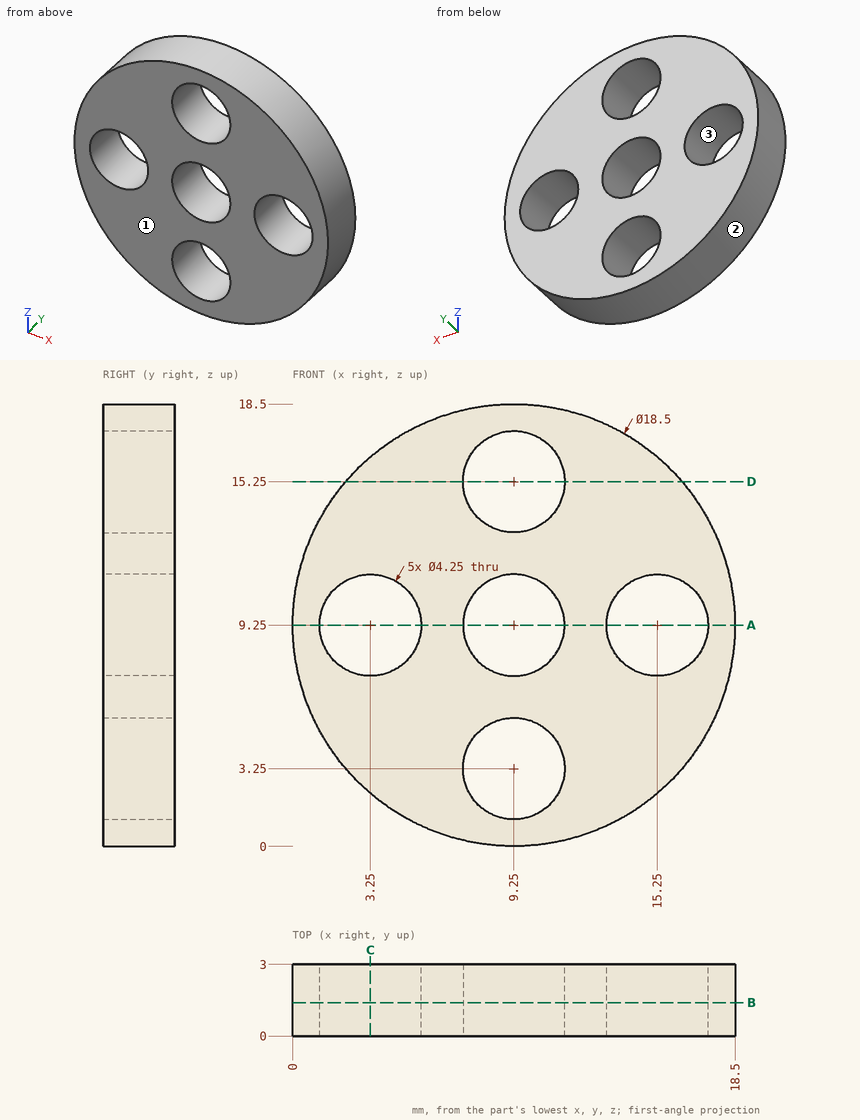
Can you work these out from the drawing? Everything is in mm from the part's minimum corner. Give positions to 0.01 mm unless a question says otherwise; leave off trailing zeros. Loops run counter-clockwise (first coordinate to the right, second up) from the corner with the lowest first, then second, coordinate; pieces in that order, holes last. Notation, with made-up numbers: (78, -15) -> (136, -15) arc R20 ccw to (136, 1) -> close; hole circle Ø5 at (61.25, 13). An arc over 180 degrees is marked (long way). Return JSON: item names as keys, results as strings.
Q1. I want a section at A-A, the plane z = 9.25. List the corners of the cut face in (x, y) for me (3 decimals), then the cut area to 4 significant figures.
Checks:
{"outline": "(0, 0) -> (1.125, 0) -> (1.125, 3) -> (0, 3) -> close; (5.375, 0) -> (7.125, 0) -> (7.125, 3) -> (5.375, 3) -> close; (11.375, 0) -> (13.125, 0) -> (13.125, 3) -> (11.375, 3) -> close; (17.375, 0) -> (18.5, 0) -> (18.5, 3) -> (17.375, 3) -> close", "area": "17.25 mm2"}
Q2. I want a section at C-C, the plane x = 3.25. List the corners of the cut face in (y, z) for me (3 decimals), then the cut area to 3 significant figures.
Checks:
{"outline": "(0, 2.21) -> (3, 2.21) -> (3, 7.125) -> (0, 7.125) -> close; (0, 11.375) -> (3, 11.375) -> (3, 16.29) -> (0, 16.29) -> close", "area": "29.5 mm2"}
Q3. I want a section at D-D, the plane z = 15.25. List the corners of the cut face in (x, y) for me (3 decimals), then the cut area to 3 significant figures.
Checks:
{"outline": "(2.21, 0) -> (7.125, 0) -> (7.125, 3) -> (2.21, 3) -> close; (11.375, 0) -> (16.29, 0) -> (16.29, 3) -> (11.375, 3) -> close", "area": "29.5 mm2"}
Q4. I want a section at B-B, the plane y = 1.4. List the corners of the cut face in (x, z) for me (3 decimals), then the cut area to 3 significant figures.
Checks:
{"outline": "circle Ø18.5 at (9.25, 9.25); hole circle Ø4.25 at (3.25, 9.25); hole circle Ø4.25 at (9.25, 3.25); hole circle Ø4.25 at (9.25, 9.25); hole circle Ø4.25 at (9.25, 15.25); hole circle Ø4.25 at (15.25, 9.25)", "area": "198 mm2"}
Q5. For pin 1 Ø5.5 at (x, z) = (3.25, 9.25) entering from +Y; pin 2 Ø2.5 at (x, z) = (9.25, 3.25) entering from -Y; pin 3 Ø1 at (y, z) = (2, 3.5) entering from +X, each with a flat end and sliding along its axis, tell me the tip position at first contact or that it passes through.
Checks:
{"pin 1": "stops at y = 3", "pin 2": "passes through", "pin 3": "stops at x = 16.87"}
Q6. We'd pull the mould along Z, two halves only. Please class the marked faces 1, 2 and 3: released by +Z, released by -Z, zero draft, split by the parting line, or undercut.
Checks:
{"face 1": "zero draft", "face 2": "split by the parting line", "face 3": "undercut"}
Q7. I need wall thicknesses on probe 1 along Z at (x, y) = (9.25, 1.2) (3 decimals); probe 2 along X at (y, z) = (2.55, 7.75); probe 3 along X at (y, z) = (1.1, 8.5). Which ranges of each line are inside material? Lowest first, please.
Checks:
{"probe 1": "z = 0 to 1.125, 5.375 to 7.125, 11.375 to 13.125, 17.375 to 18.5", "probe 2": "x = 0.12 to 1.74, 4.76 to 7.74, 10.76 to 13.74, 16.76 to 18.38", "probe 3": "x = 0.03 to 1.26, 5.24 to 7.26, 11.24 to 13.26, 17.24 to 18.47"}
